Check sheet for the modelled part. Datum: model origin and axes. Units: mm. Face numbers are marked on the shaded views. A direction names the side the tool comes from. Give positions to 0.01 mm unless a question says otherwise; leave off trailing zeros. Write each loop counter-clockwise with the first axis right and the second up, starting at its lowest first coordinate (ties: lowest second). Pieces come first, ordered by that corner, then holes. Notation, with made-up numbers: (-26.75, 32) -> (-1.75, 32) arc R12 cw to (-1.75, 39) -> close; hole circle Ø10 at (65, -33). An arc over 180 degrees is marked (long way). Use a Markdown table: item, result. Add a question column.
1. Cross-section at C-C (y = -8.25). Enter the section's corners in (x, z).
2. Release check for a two-part mould opening along X. For the marked faces 3, 4 and 5 record: released by +X, released by -X, zero draft, split by the parting line, or undercut.
3. Gauge pin test, flat ends, axial feed: P1, Ø7, axis at x = 0, z = -6, coming from the -Y side; P2, Ø3, axis at x = 1.5, z = -5.5, coming from the -Y side; P3, Ø3, axis at x = -5.5, y = 0.5, coming from the +Z side; P4, Ø6, axis at y = 0, z = -6, coming from the +X side. Record the tip position at first contact, or that the pin passes through.
4. Scan lines: probe 1 along Z at (x, y) = (0, 7.9); probe 2 along Y at (x, z) = (-3, -6.5); probe 3 along Y at (x, z) = (0.25, 1). Record each from-to range of solid material in increasing order. Write a range as [from, to].
5. Cross-section at B-B (x = 0). Enter the section's corners in (y, z), then the cut area to 3 significant figures.
6. Cross-section at A-A (x = -2.75). Enter the section's corners in (y, z), then the cut area to 3 significant figures.
7. Cross-section at D-D (z = -6). Enter the section's corners in (x, y), then the cut area to 3 significant figures.
8. Set-up check for the marked faces 1 and 2: record each of +Z, -Z, +X, -X, +Y, -Y from which the full face is reachable in a straight line by a thin tool's end or side.
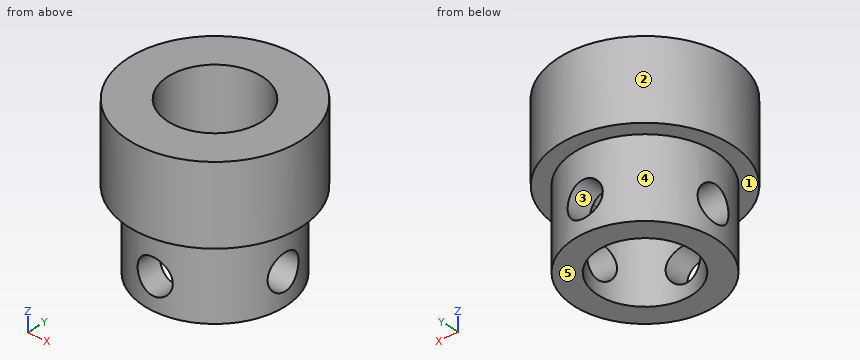
from build123d import *

# Parameters (mm, degrees)
ESQUISSE1_R                = 11
ESQUISSE1_R_2              = 6
BOSS_EXTRU_1_DEPTH         = 10
ESQUISSE2_R                = 9
ESQUISSE2_R_2              = 6
BOSS_EXTRU_2_DEPTH         = 10
D_GAGEMENT_M41_D           = 4.5
D_GAGEMENT_M41_ON_FACE_2_D = 4.5


with BuildPart() as part:
    # Esquisse1 → Boss.-Extru.1 (new body)
    with BuildSketch(Plane.XY):
        Circle(ESQUISSE1_R)
        Circle(ESQUISSE1_R_2, mode=Mode.SUBTRACT)
    extrude(amount=BOSS_EXTRU_1_DEPTH)

    # Esquisse2 → Boss.-Extru.2 (add)
    with BuildSketch(Plane(origin=(0, 0, 0), x_dir=(-1, 0, 0), z_dir=(0, 0, -1))):
        Circle(ESQUISSE2_R)
        Circle(ESQUISSE2_R_2, mode=Mode.SUBTRACT)
    extrude(amount=BOSS_EXTRU_2_DEPTH)

    # Dégagement M41 (through all)
    with Locations(Plane(origin=(0, 9, -6), x_dir=(1, 0, 0), z_dir=(0, 1, 0))):
        with Locations((0, 0)):
            Hole(D_GAGEMENT_M41_D / 2)

    # Dégagement M41 on face 2 (through all)
    with Locations(Plane(origin=(-9, 0, -6), x_dir=(0, 0, -1), z_dir=(-1, 0, 0))):
        with Locations((0, 0)):
            Hole(D_GAGEMENT_M41_ON_FACE_2_D / 2)


solid = part.part
Worked answers:
| question | item | result |
|---|---|---|
| 1 | outline | (-7.28, 0) -> (-3.6, 0) -> (-3.6, -10) -> (3.6, -10) -> (3.6, 0) -> (7.28, 0) -> (7.28, 10) -> (-7.28, 10) -> close; hole circle Ø4.5 at (0, -6) |
| 2 | face 3 | undercut |
| 2 | face 4 | split by the parting line |
| 2 | face 5 | zero draft |
| 3 | P1 | stops at y = -9 |
| 3 | P2 | stops at y = -8.93 |
| 3 | P3 | stops at z = 10 |
| 3 | P4 | stops at x = 9 |
| 4 | probe 1 | z = [-10, -8.25], [-3.75, 10] |
| 4 | probe 2 | y = [-8.49, -5.2], [5.2, 8.49] |
| 4 | probe 3 | y = [-11, -5.99], [5.99, 11] |
| 5 | outline | (-11, 0) -> (-9, 0) -> (-9, -3.75) -> (-6, -3.75) -> (-6, 10) -> (-11, 10) -> close; (-9, -10) -> (-6, -10) -> (-6, -8.25) -> (-9, -8.25) -> close; (6, -10) -> (9, -10) -> (9, -8.25) -> (6, -8.25) -> close; (6, -3.75) -> (9, -3.75) -> (9, 0) -> (11, 0) -> (11, 10) -> (6, 10) -> close |
| 5 | area | 133 mm² |
| 6 | outline | (-10.65, 0) -> (-8.57, 0) -> (-8.57, -10) -> (-5.33, -10) -> (-5.33, 10) -> (-10.65, 10) -> close; (5.33, -10) -> (8.57, -10) -> (8.57, 0) -> (10.65, 0) -> (10.65, 10) -> (5.33, 10) -> close |
| 6 | area | 171 mm² |
| 7 | outline | (-8.71, -2.25) arc R9 ccw to (-2.25, -8.71) -> (-2.25, -5.56) arc R6 cw to (-5.56, -2.25) -> close; (-8.71, 2.25) -> (-5.56, 2.25) arc R6 cw to (-2.25, 5.56) -> (-2.25, 8.71) arc R9 ccw to start; (2.25, -8.71) arc R9 ccw to (8.71, -2.25) -> (5.56, -2.25) arc R6 cw to (2.25, -5.56) -> close; (2.25, 5.56) arc R6 cw to (5.56, 2.25) -> (8.71, 2.25) arc R9 ccw to (2.25, 8.71) -> close |
| 7 | area | 86.5 mm² |
| 8 | face 1 | -Z |
| 8 | face 2 | +Z, -Z |
